Model file for the job. Use its own axes, mm. A direction names the side the tool comes from. Round coordinates to 2 decimals unless told otherwise and drop trailing zeros. Loops run counter-clockwise (first coordinate to the right, second up) from the corner with the lowest first, then second, coordinate; pieces in that order, holes last. Notation, with made-up numbers: (-37.5, 12) -> (-11.5, 12) arc R13 ccw to (-11.5, 30) -> close; hole circle Ø8 at (2.25, 84). An arc over 180 degrees is marked (long way). Use a Markdown table: item, result. Add a question column.
```python
from build123d import *

# Parameters (mm, degrees)
SKETCH1_R           = 21.6
SKETCH1_R_2         = 20
BOSS_EXTRUDE1_DEPTH = 10
BOSS_EXTRUDE2_START = -6
SKETCH1_3_R         = 21.6
SKETCH1_3_R_2       = 20
SKETCH1_3_R_3       = 10
SKETCH1_3_R_4       = 1.6
BOSS_EXTRUDE2_DEPTH = 6
SKETCH1_5_R         = 1.6
CUT_EXTRUDE2_DEPTH  = 33.14218412
CUT_EXTRUDE1_START  = -6
CUT_EXTRUDE1_DEPTH  = 3
BOSS_EXTRUDE3_START = -2.8
SKETCH1_6_R         = 1.6
BOSS_EXTRUDE3_DEPTH = 0.2
CIRPATTERN2_COUNT   = 2
SKETCH3_R           = 1.6
CUT_EXTRUDE4_DEPTH  = 33.14218412
SKETCH3_3_R         = 1.6
CUT_EXTRUDE5_DEPTH  = 3
CIRPATTERN3_COUNT   = 2


with BuildPart() as part:
    # Sketch1 → Boss-Extrude1 (new body)
    with BuildSketch(Plane(origin=(0, 0, 0), x_dir=(1, 0, 0), z_dir=(0, 1, 0))):
        with Locations(Location((0, 0, 0), (0, 0, 270))):
            Circle(SKETCH1_R)
        with Locations(Location((0, 0, 0), (0, 0, 270))):
            Circle(SKETCH1_R_2, mode=Mode.SUBTRACT)
    extrude(amount=BOSS_EXTRUDE1_DEPTH)

    # Sketch1<3> → Boss-Extrude2 (add)
    # profile 1 of 4: a face of its own
    with BuildSketch(Plane(origin=(0, 0, 0), x_dir=(1, 0, 0), z_dir=(0, 1, 0)).offset(BOSS_EXTRUDE2_START)):
        with Locations(Location((0, 0, 0), (0, 0, 270))):
            Circle(SKETCH1_3_R)
        with Locations(Location((0, 0, 0), (0, 0, 270))):
            Circle(SKETCH1_3_R_2, mode=Mode.SUBTRACT)
    # profile 2 of 4: a face of its own
    with BuildSketch(Plane(origin=(0, 0, 0), x_dir=(1, 0, 0), z_dir=(0, 1, 0)).offset(BOSS_EXTRUDE2_START)):
        with Locations(Location((0, 0, 0), (0, 0, 270))):
            Circle(SKETCH1_3_R_2)
        with Locations(Location((0, 0, 0), (0, 0, 270))):
            Circle(SKETCH1_3_R_3, mode=Mode.SUBTRACT)
        Polygon((10.271761873, 11.432595565), (10.234009445, 14.78101431), (7.315317535, 16.42252912), (4.434378054, 14.715625186), (4.472130483, 11.367206441), (7.390822392, 9.725691631), align=None, mode=Mode.SUBTRACT)
    # profile 3 of 4: a face of its own
    with BuildSketch(Plane(origin=(0, 0, 0), x_dir=(1, 0, 0), z_dir=(0, 1, 0)).offset(BOSS_EXTRUDE2_START)):
        Polygon((7.390822392, 9.725691631), (10.271761873, 11.432595565), (10.234009445, 14.78101431), (7.315317535, 16.42252912), (4.434378054, 14.715625186), (4.472130483, 11.367206441), align=None)
        with Locations((7.353069964, 13.074110375)):
            Circle(SKETCH1_3_R_4, mode=Mode.SUBTRACT)
    # profile 4 of 4: a face of its own
    with BuildSketch(Plane(origin=(0, 0, 0), x_dir=(1, 0, 0), z_dir=(0, 1, 0)).offset(BOSS_EXTRUDE2_START)):
        with Locations((7.353069964, 13.074110375)):
            Circle(SKETCH1_3_R_4)
    extrude(amount=BOSS_EXTRUDE2_DEPTH)

    # Sketch1<5> → Cut-Extrude2 (cut, through all)
    with BuildSketch(Plane(origin=(0, 0, 0), x_dir=(1, 0, 0), z_dir=(0, 1, 0))):
        with Locations(Location((7.353069964, 13.074110375, 0), (0, 0, 270))):
            Circle(SKETCH1_5_R)
    cut_extrude2 = extrude(amount=-CUT_EXTRUDE2_DEPTH, mode=Mode.SUBTRACT)

    # Sketch1<4> → Cut-Extrude1 (cut)
    with BuildSketch(Plane(origin=(0, 0, 0), x_dir=(1, 0, 0), z_dir=(0, 1, 0)).offset(CUT_EXTRUDE1_START)):
        Polygon((10.234009445, 14.78101431), (7.315317535, 16.42252912), (4.434378054, 14.715625186), (4.472130483, 11.367206441), (7.390822392, 9.725691631), (10.271761873, 11.432595565), align=None)
    cut_extrude1 = extrude(amount=CUT_EXTRUDE1_DEPTH, mode=Mode.SUBTRACT)

    # Sketch1<6> → Boss-Extrude3 (add)
    with BuildSketch(Plane(origin=(0, 0, 0), x_dir=(1, 0, 0), z_dir=(0, 1, 0)).offset(BOSS_EXTRUDE3_START)):
        with Locations(Location((7.353069964, 13.074110375, 0), (0, 0, 270))):
            Circle(SKETCH1_6_R)
    boss_extrude3 = extrude(amount=-BOSS_EXTRUDE3_DEPTH)

    # CirPattern2: Cut-Extrude2, Cut-Extrude1, Boss-Extrude3 ×2 about axis
    cirpattern2_axis = Axis((0, 0, 0), (0, 1, 0))
    add([cut_extrude2.rotate(cirpattern2_axis, i * 360 / CIRPATTERN2_COUNT) for i in range(1, CIRPATTERN2_COUNT)], mode=Mode.SUBTRACT)
    add([cut_extrude1.rotate(cirpattern2_axis, i * 360 / CIRPATTERN2_COUNT) for i in range(1, CIRPATTERN2_COUNT)], mode=Mode.SUBTRACT)
    add([boss_extrude3.rotate(cirpattern2_axis, i * 360 / CIRPATTERN2_COUNT) for i in range(1, CIRPATTERN2_COUNT)])

    # Sketch3 → Cut-Extrude4 (cut, through all)
    with BuildSketch(Plane(origin=(0, 0, 0), x_dir=(1, 0, 0), z_dir=(0, 1, 0))):
        with Locations(Location((13.074110375, -7.353069964, 0), (0, 0, 270))):
            Circle(SKETCH3_R)
    cut_extrude4 = extrude(amount=-CUT_EXTRUDE4_DEPTH, mode=Mode.SUBTRACT)

    # Sketch3<3> → Cut-Extrude5 (cut)
    with BuildSketch(Plane(origin=(0, 0, 0), x_dir=(1, 0, 0), z_dir=(0, 1, 0))):
        Polygon((14.715625186, -4.434378054), (11.367206441, -4.472130483), (9.725691631, -7.390822392), (11.432595565, -10.271761873), (14.78101431, -10.234009445), (16.42252912, -7.315317535), align=None)
        with Locations(Location((13.074110375, -7.353069964, 0), (0, 0, 270))):
            Circle(SKETCH3_3_R, mode=Mode.SUBTRACT)
    cut_extrude5 = extrude(amount=-CUT_EXTRUDE5_DEPTH, mode=Mode.SUBTRACT)

    # CirPattern3: Cut-Extrude4, Cut-Extrude5 ×2 about axis
    cirpattern3_axis = Axis((0, 0, 0), (0, 1, 0))
    add([cut_extrude4.rotate(cirpattern3_axis, i * 360 / CIRPATTERN3_COUNT) for i in range(1, CIRPATTERN3_COUNT)], mode=Mode.SUBTRACT)
    add([cut_extrude5.rotate(cirpattern3_axis, i * 360 / CIRPATTERN3_COUNT) for i in range(1, CIRPATTERN3_COUNT)], mode=Mode.SUBTRACT)


solid = part.part
```
1) Cut at A-A on x = 0. Write the cut outline in (y, z).
2) Cut at C-C on y = 7.5. Write the cut outline in (x, z), and give its area (3 significant figures).
3) Cut at D-D on x = 17. Write the cut outline in (y, z), and give its area (3 significant figures).
4) Pin check, flat tips, straight feed: pin 1 Ø8 at (y, z) = (7, 7) entering from +X; pin 2 Ø5 at (x, z) = (10.5, -13) entering from +Y; pin 3 Ø3 at (x, z) = (-7.35, 13.07) entering from -Y; pin 4 Ø4.5 at (x, z) = (-6, 14) entering from -Y. Stop position of each tip, or through.
5) Wall check: probe 1 along X at (y, z) = (-1.25, 0.5); probe 2 along X at (y, z) = (-4, 6.5); probe 3 along Y at (x, z) = (12, 15). Give the ranges that are in metal, low to high. Write a range as from..to.
6) Pull direction Z, two halves, no side cores. Call faces 4 (the face through (-14.3, 10, 14.3)), 5 (the face through (6.5, 1.9, 20.6)), 6 (the face through (-15.581, -1.479, -5.895)): +Z half, -Z half, draft (parallel to the pull), parting line (faces both ways), or undercut.
7) Cut at B-B on z = 0. Write the cut outline in (x, y), and give its area (3 significant figures).
8) Tool access for faces 1 (the face through (-8.795, -4.521, 15.59)), 2 (the face through (-11.51, -4.48, -7.01)), 3 (the face through (7, -2.8, -13)): list every direction of +Z, -Z, +X, -X, +Y, -Y with a clear straight run to the whole face (end or side of a thin tool).
Established:
| question | item | result |
|---|---|---|
| 1 | outline | (-6, -21.6) -> (10, -21.6) -> (10, -20) -> (0, -20) -> (0, -10) -> (-6, -10) -> close; (-6, 10) -> (0, 10) -> (0, 20) -> (10, 20) -> (10, 21.6) -> (-6, 21.6) -> close |
| 2 | outline | circle Ø43.2 at (0, 0); hole circle Ø40 at (0, 0) |
| 2 | area | 209 mm^2 |
| 3 | outline | (-6, -13.33) -> (10, -13.33) -> (10, -10.54) -> (0, -10.54) -> (0, 10.54) -> (10, 10.54) -> (10, 13.33) -> (-6, 13.33) -> close |
| 3 | area | 216 mm^2 |
| 4 | pin 1 | stops at x = 21.39 |
| 4 | pin 2 | stops at y = 0 |
| 4 | pin 3 | stops at y = -3 |
| 4 | pin 4 | stops at y = -6 |
| 5 | probe 1 | x = -21.59..-9.99, 9.99..21.59 |
| 5 | probe 2 | x = -20.6..-7.6, 7.6..11.72, 14.43..20.6 |
| 5 | probe 3 | y = -6..0 |
| 6 | face 4 | draft |
| 6 | face 5 | parting line |
| 6 | face 6 | undercut |
| 7 | outline | (-21.6, -6) -> (-10, -6) -> (-10, 0) -> (-20, 0) -> (-20, 10) -> (-21.6, 10) -> close; (10, -6) -> (21.6, -6) -> (21.6, 10) -> (20, 10) -> (20, 0) -> (10, 0) -> close |
| 7 | area | 171 mm^2 |
| 8 | face 1 | -Y |
| 8 | face 2 | +Y, -Y |
| 8 | face 3 | +Y |
